from build123d import *

# Parameters (mm, degrees)
F1_DEPTH = 10
F3_DEPTH = 5.1961524227


with BuildPart() as f1:
    # F0 (on Top) → F1 (new body)
    with BuildSketch(Plane.XY):
        Polygon((-1.3409011788, -2.6836512495), (1.6536595675, -2.5030801095), (2.9945607463, 0.18057114), (1.3409011788, 2.6836512495), (-1.6536595675, 2.5030801095), (-2.9945607463, -0.18057114), align=None)
    extrude(amount=F1_DEPTH)

    # F2 (on face) → F3 (cut, through all)
    with BuildSketch(Plane(origin=(0.1563791944, -2.5933656795, 0), x_dir=(0.9981869154, 0.06019038, 0), z_dir=(0.06019038, -0.9981869154, 0))):
        with BuildLine():
            ThreePointArc((-1.5, 5), (0, 3.5), (1.5, 5))
            ThreePointArc((1.5, 5), (0, 6.5), (-1.5, 5))
        make_face()
    extrude(amount=-F3_DEPTH, mode=Mode.SUBTRACT)


solid = f1.part
The listing builds one solid part. Answer for the finished solid, in the listing's coordinates (mm). Coordinates: 2 decimals unless noted, no trailing zeros. Write each loop counter-clockwise with the first axis right and the second up, starting at its lowest first coordinate (ties: lowest second). Pieces come first, ordered by that corner, then holes. Notation, with made-up numbers: (61, -1.5) -> (112, -1.5) arc R29 cw to (112, 20.5) -> close; hole circle Ø2 at (41, -8). An arc over 180 degrees is marked (long way). One line per question, with ' | ' between items.
1. Straight lines are drawn through the part: line 1 (Z direction, x = -0.1, y = 0.85); line 2 (X direction, y = -1.8, z = 5); line 3 (Z direction, x = -1.05, y = 2.3). For each, find the intervals that lie inside material, in ascending order.
Verdict:
line 1: z = 0 to 3.5, 6.5 to 10 | line 2: x = -1.92 to -1.39, 1.61 to 2 | line 3: z = 0 to 3.81, 6.19 to 10
2. Section D-D (x = -2.2) is taken. Determine the outline of the cut face in (y, z), and give its area (3 significant figures).
Verdict:
outline: (-1.38, 0) -> (1.41, 0) -> (1.41, 10) -> (-1.38, 10) -> close | area: 27.9 mm^2
3. Given pin 1 Ø1.5 at (x, z) = (0.5, 9) entering from +Y; pin 2 Ø3 at (x, z) = (1.5, 3) entering from -Y, each flat-ended and moving along its own axis, determine where each tip first touches the part or whether it passes through.
Verdict:
pin 1: stops at y = 2.68 | pin 2: stops at y = -2.6
4. Section B-B (z = 8.5) is taken. Determine the outline of the cut face in (x, y).
Verdict:
outline: (-2.99, -0.18) -> (-1.34, -2.68) -> (1.65, -2.5) -> (2.99, 0.18) -> (1.34, 2.68) -> (-1.65, 2.5) -> close
5. For a pull along X with two mould halves and no side action, classify faces 1 (the flat face through (2.315, -1.18, 4.93)), 2 (the flat face through (-2.18, -1.41, 4.93)), 3 (the cylindrical face through (0.69, 0.01, 3.67)) as released by +X, released by -X, zero draft, split by the parting line, or undercut.
Verdict:
face 1: released by +X | face 2: released by -X | face 3: undercut
6. Section C-C (x = 2.45) is taken. Determine the outline of the cut face in (y, z), and give its area (3 significant figures).
Verdict:
outline: (-0.91, 0) -> (1, 0) -> (1, 10) -> (-0.91, 10) -> close | area: 19.1 mm^2
7. Section A-A (z = 4.5) is taken. Determine the outline of the cut face in (x, y), and give its area (3 significant figures).
Verdict:
outline: (-2.99, -0.18) -> (-1.34, -2.68) -> (-1.26, -2.68) -> (-1.57, 2.51) -> (-1.65, 2.5) -> close; (1.26, 2.68) -> (1.57, -2.51) -> (1.65, -2.5) -> (2.99, 0.18) -> (1.34, 2.68) -> close | area: 8.69 mm^2
